The drawing under review shows one solid part. Ordinate dimensions are in mm from its lowest x, y, z. Coordinates: 2 decimals unless noted, no trailing zeros. Write each loop counter-clockwise with the first axis right and the second up, starting at its lowest first coordinate (ties: lowest second). Pieces come first, ordered by that corner, then holes. Notation, with made-up numbers: M 29.5,-23 L 86.5,-23 A33 cw 86.5,9 Z; hole C 37,83.5 d9. An arc over 180 degrees is marked long. Write item = value, one per line.
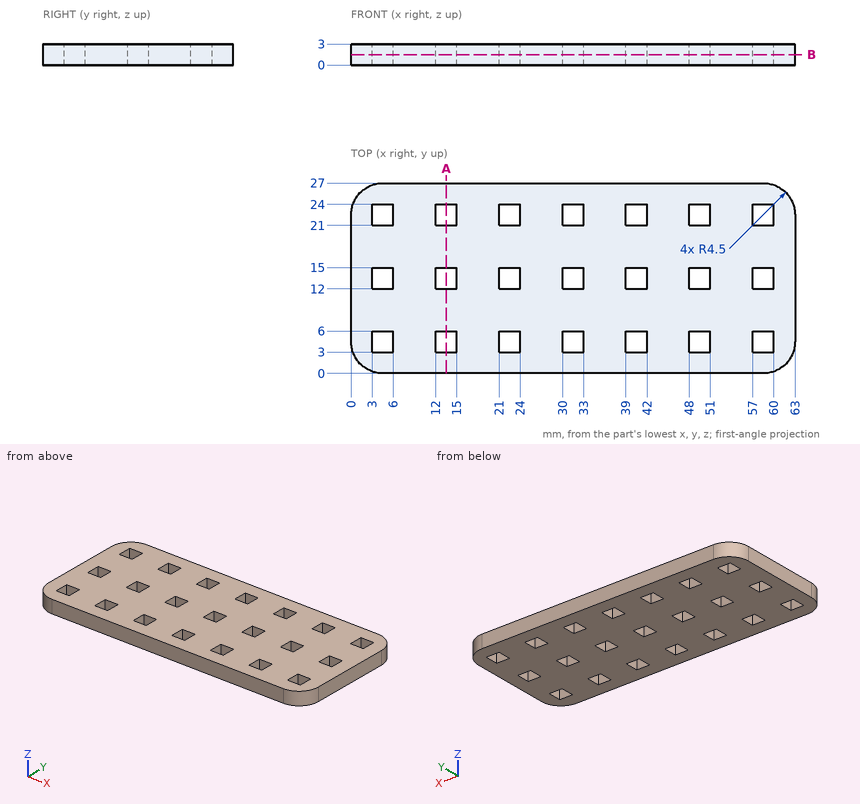
Q1. Wall thickness on line 1 (Y direction, x = 31, z = 1); line 2 (X direction, y = 1, z = 0.8); line 3 (X direction, y = 2, z = 2.65): over which ranges is each line inside the solid? List them lowest first.
Check result:
line_1 = 0 to 3, 6 to 12, 15 to 21, 24 to 27
line_2 = 1.67 to 61.33
line_3 = 0.76 to 62.24
Q2. Consider section B-B, the plane z = 1.5. State how many separate pieces and enclosed holes the cut face has, and give its area (3 significant figures).
Check result:
separate_pieces = 1
enclosed_holes = 21
area = 1,490 mm²
Q3. For P1, Ø1.5, axis at y = 23, z = 1, coming from the -X side, flat-tipped, find the tip position at first contact; note if it passes through.
Check result:
P1 = 0
Q4. Consider section A-A, the plane x = 13.5. State the section outline as (y, z) points, and give its area (3 significant figures).
Check result:
outline = M 0,0 L 3,0 L 3,3 L 0,3 Z; M 6,0 L 12,0 L 12,3 L 6,3 Z; M 15,0 L 21,0 L 21,3 L 15,3 Z; M 24,0 L 27,0 L 27,3 L 24,3 Z
area = 54.0 mm²
